```python
from build123d import *

# Parameters (mm, degrees)
F3_DEPTH = 0.508


with BuildPart() as f1:
    # F0 (on Right) → F1 (revolve)
    with BuildSketch(Plane.YZ):
        Polygon((12.7, 7.128853), (0, 4.8895), (0, 4.5085), (12.7, 4.5085), align=None)
    revolve(axis=Axis((0, 6.35, 0), (0, 1, 0)))

    # F2 (on Top) → F3 (cut, symmetric)
    with BuildSketch(Plane.XY):
        Polygon((15.353079, 15.146448), (1.846084, 15.401297), (1.846084, 0), (15.353079, 0), align=None)
    extrude(amount=F3_DEPTH, both=True, mode=Mode.SUBTRACT)


solid = f1.part
```
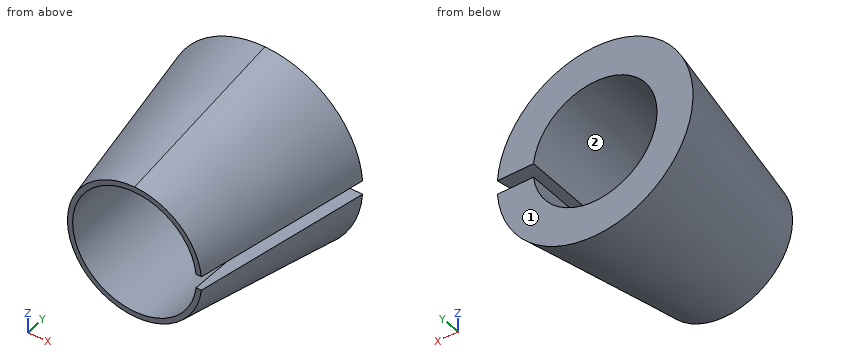
Verification items for the finished model (mm, model axes). Face numbers are marked on the shaded views. Coordinates: 2 decimals unless noted, no trailing zeros. Order: outer loops, then holes, each group sorted by start corner. A loop starts at its lowest first (then second) coordinate and runs counter-clockwise, first axis right, second up. Notation, with made-up numbers: (-27, 30) -> (-3, 30) arc R25 cw to (-3, 59) -> close; hole circle Ø6 at (83, -11). An arc over 180 degrees is marked (long way). Put each result on its own line as item: value. Start each with the question number.
1) Go/stop test with flat-tipped pins: pin 1 (1.3 mm diameter, centred on x = 6, y = 7, fed in from -Z); pin 2 (1 mm diameter, centred on y = 5.5, z = 1, fed in from +X); pin 3 (1.5 mm diameter, centred on x = 1.5, y = 11, fed in from -Z). Record where each tip stops, or that it passes through.
2) Material ranges on L1, parallel to Z at x = -4, y = 5; L2, parallel to Z at x = 0, y = 6; L3, parallel to X at y = 5.5, z = -1.5, recorded low to high.
3) Release check for a two-part mould opening along Z. For the marked faces 1 and 2 record: pulls with the +Z half, pulls with the -Z half, needs draft (parallel to the pull), parting line crosses it, or undercut.
4) Cross-section at B-B (y = 9). Enter the section's corners in (x, z), plus the area to 3 significant figures.
5) Cross-section at A-A (z = 0). Enter the section's corners in (x, y).
Geometry check:
1. pin 1: stops at z = -3
1. pin 2: stops at x = 5.89
1. pin 3: stops at z = -6.86
2. L1: z = -4.16 to -2.08, 2.08 to 4.16
2. L2: z = -5.95 to -4.51, 4.51 to 5.95
2. L3: x = -5.66 to -4.25, 4.25 to 5.66
3. face 1: needs draft
3. face 2: undercut
4. outline: (4.48, -0.51) arc R4.51 cw (long way) to (4.48, 0.51) -> (6.46, 0.51) arc R6.48 ccw (long way) to (6.46, -0.51) -> close
4. area: 65.9 mm^2
5. outline: (-7.13, 12.7) -> (-4.89, 0) -> (-4.51, 0) -> (-4.51, 12.7) -> close
